Verification items for the finished model (mm, model axes). A direction names the side the tool comes from. Round coordinates to 2 decimals unless told otherwise and drop trailing zeros. Loops run counter-clockwise (first coordinate to the right, second up) from the corner with the lowest first, then second, coordinate; pieces in that order, holes last. Notation, with made-up numbers: M 60.5,7 L 109.5,7 A12 cw 109.5,14 Z; hole C 55.5,-35.5 d8. An arc over 180 degrees is marked long. Write item = value, one per line. Start each with the question number.
from build123d import *

# Parameters (mm, degrees)
SKETCH_1_R          = 5
EXTRUDE_1_DEPTH     = 10
SKETCH_2_R          = 1.25
CUT_EXTRUDE_1_DEPTH = 10


with BuildPart() as part:
    # 草图1 → 凸台-拉伸1 (new body)
    with BuildSketch(Plane.XY):
        with BuildLine():
            Line((-50, 10), (50, 10))
            ThreePointArc((50, 10), (60, 0), (50, -10))
            Line((50, -10), (-50, -10))
            ThreePointArc((-50, -10), (-60, 0), (-50, 10))
        make_face()
        with Locations((50, 0)):
            Circle(SKETCH_1_R, mode=Mode.SUBTRACT)
        with BuildLine():
            Line((-53, 4), (-47, 4))
            ThreePointArc((-47, 4), (-50, -5), (-53, 4))
        make_face(mode=Mode.SUBTRACT)
    extrude(amount=EXTRUDE_1_DEPTH)

    # 草图2 → 切除-拉伸1 (cut)
    with BuildSketch(Plane.XZ.offset(10)):
        with Locations((-50, 5)):
            Circle(SKETCH_2_R)
    extrude(amount=-CUT_EXTRUDE_1_DEPTH, mode=Mode.SUBTRACT)


solid = part.part
1. Mould release check, pull along Y, two halves, no side actions. Record for faces 3 (the flat face through (1, -10, 5)), 4 (the flat face through (-1, 10, 5)), 5 (the cylindrical face through (-49.423, -7.454, 3.891)), 6 (the cylindrical face through (45, 0, 5)): pulls with the +Y half, pulls with the -Y half, needs draft (parallel to the pull), parting line crosses it, or undercut.
2. Tool access check on faces 1 (the cylindrical face through (60, 0, 5)), 2 (the flat face through (-50, 4, 5)). Record the directions out of +Z, -Z, +X, -X, +Y, -Y that give a thin tool (end or side, any length) a straight path to the whole face; none if there is none.
3. Section check B-B, the plane z = 2. Enter the section's corners in (x, y).
4. Thickness scan on line 1 (Y direction, x = 50, z = 6.25); line 2 (X direction, y = 1.25, z = 3); line 3 (Y direction, x = -50, z = 2.5). Record the ranges inside material, lowest first.
5. Section check A-A, the plane y = 0. Enter the section's corners in (x, z).
6. Gauge pin test, flat ends, axial feed: P1, Ø1.5, axis at y = 2, z = 2.5, coming from the -X side; P2, Ø1.5, axis at y = 3.5, z = 7.5, coming from the -X side. Record the tip position at first contact, or that the pin passes through.
Computed values:
q1.face_3 = pulls with the -Y half
q1.face_4 = pulls with the +Y half
q1.face_5 = needs draft
q1.face_6 = undercut
q2.face_1 = +Z, -Z, +X
q2.face_2 = +Z, -Z
q3.outline = M -50,-10 L 50,-10 A10 ccw 50,10 L -50,10 A10 ccw Z; hole M -53,4 A5 ccw long -47,4 Z; hole C 50,0 d10
q4.line_1 = -10 to -5, 5 to 10
q4.line_2 = -59.92 to -54.84, -45.16 to 45.16, 54.84 to 59.92
q4.line_3 = -10 to -5, 4 to 10
q5.outline = M -60,0 L -55,0 L -55,10 L -60,10 Z; M -45,0 L 45,0 L 45,10 L -45,10 Z; M 55,0 L 60,0 L 60,10 L 55,10 Z
q6.P1 = -59.92
q6.P2 = -59.61
